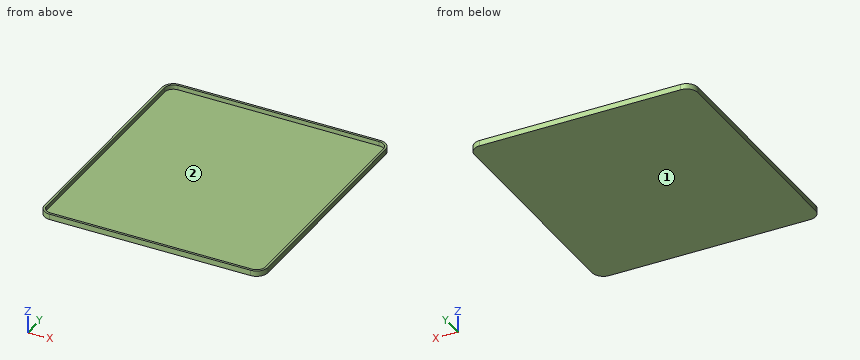
from build123d import *

# Parameters (mm, degrees)
F1_DEPTH = 0.5
F3_DEPTH = 2


with BuildPart() as f1:
    # F0 (on Top) → F1 (new body)
    with BuildSketch(Plane.XY):
        with BuildLine():
            Line((-45, -53.918237), (45, -53.918237))
            ThreePointArc((45, -53.918237), (48.535534, -52.453771), (50, -48.918237))
            Line((50, -48.918237), (50, 51.081763))
            ThreePointArc((50, 51.081763), (48.535534, 54.617297), (45, 56.081763))
            Line((45, 56.081763), (-45, 56.081763))
            ThreePointArc((-45, 56.081763), (-48.535534, 54.617297), (-50, 51.081763))
            Line((-50, 51.081763), (-50, -48.918237))
            ThreePointArc((-50, -48.918237), (-48.535534, -52.453771), (-45, -53.918237))
        make_face()
    extrude(amount=F1_DEPTH)

    # F2 (on face) → F3 (join)
    with BuildSketch(Plane.XY.offset(0.5)):
        with BuildLine():
            ThreePointArc((45, -53.918237), (48.535534, -52.453771), (50, -48.918237))
            Line((50, -48.918237), (50, 51.081763))
            ThreePointArc((50, 51.081763), (48.535534, 54.617297), (45, 56.081763))
            Line((45, 56.081763), (-45, 56.081763))
            ThreePointArc((-45, 56.081763), (-48.535534, 54.617297), (-50, 51.081763))
            Line((-50, 51.081763), (-50, -48.918237))
            ThreePointArc((-50, -48.918237), (-48.535534, -52.453771), (-45, -53.918237))
            Line((-45, -53.918237), (45, -53.918237))
        make_face()
        with BuildLine():
            Line((49, 51.081763), (49, -48.918237))
            ThreePointArc((49, -48.918237), (47.828427, -51.746664), (45, -52.918237))
            Line((45, -52.918237), (-45, -52.918237))
            ThreePointArc((-45, -52.918237), (-47.828427, -51.746664), (-49, -48.918237))
            Line((-49, -48.918237), (-49, 51.081763))
            ThreePointArc((-49, 51.081763), (-47.828427, 53.91019), (-45, 55.081763))
            Line((-45, 55.081763), (45, 55.081763))
            ThreePointArc((45, 55.081763), (47.828427, 53.91019), (49, 51.081763))
        make_face(mode=Mode.SUBTRACT)
    extrude(amount=F3_DEPTH)


solid = f1.part
Geometry check sheet. Reference: the model listing, model coordinates, mm. Face numbers are marked on the shaded views. Round coordinates to 2 decimals unless told otherwise and drop trailing zeros. Order: outer loops, then holes, each group sorted by start corner. A loop starts at its lowest first (then second) coordinate and runs counter-clockwise, first axis right, second up. Notation, with made-up numbers: M -14.5,25 L -9.5,25 A23 cw -9.5,59 Z; hole C 58,-26.5 d4. An arc over 180 degrees is marked long. Answer in a Markdown table with one row per item.
(1) Scan lines: probe 1 along X at (y, z) = (23, 1.5); probe 2 along Y at (x, z) = (-30.5, 1.4); probe 3 along Z at (x, y) = (18, 40). Record each from-to range of solid material in increasing order. Write a range as from..to.
Responses:
| item | result |
|---|---|
| probe 1 | x = -50..-49, 49..50 |
| probe 2 | y = -53.92..-52.92, 55.08..56.08 |
| probe 3 | z = 0..0.5 |
(2) Sectioned sample at A-A, the plane z = 1.9. Record the cut outline in (x, y), and give its area (3 significant figures).
Responses:
| item | result |
|---|---|
| outline | M -50,-48.92 A5 ccw -45,-53.92 L 45,-53.92 A5 ccw 50,-48.92 L 50,51.08 A5 ccw 45,56.08 L -45,56.08 A5 ccw -50,51.08 Z; hole M -49,-48.92 A4 ccw -45,-52.92 L 45,-52.92 A4 ccw 49,-48.92 L 49,51.08 A4 ccw 45,55.08 L -45,55.08 A4 ccw -49,51.08 Z |
| area | 408 mm² |
(3) Sectioned sample at B-B, the plane y = 47.5. Record the cut outline in (x, z), and give its area (3 significant figures).
Responses:
| item | result |
|---|---|
| outline | M -50,0 L 50,0 L 50,2.5 L 49,2.5 L 49,0.5 L -49,0.5 L -49,2.5 L -50,2.5 Z |
| area | 54.0 mm² |
(4) Sectioned sample at C-C, the plane x = 17. Record the cut outline in (y, z), and give its area (3 significant figures).
Responses:
| item | result |
|---|---|
| outline | M -53.92,0 L 56.08,0 L 56.08,2.5 L 55.08,2.5 L 55.08,0.5 L -52.92,0.5 L -52.92,2.5 L -53.92,2.5 Z |
| area | 59.0 mm² |
(5) Draft check along Y on the marked faces 1 and 2. Enter one of: released by +Y, released by -Y, zero draft, split by the parting line, or undercut.
Responses:
| item | result |
|---|---|
| face 1 | zero draft |
| face 2 | undercut |
(6) Go/stop test with flat-tipped pins: P1, Ø4, axis at x = 29.5, y = 8, coming from the +Z side; P2, Ø12, axis at x = 40, y = -14.5, coming from the -Z side. Record where each tip stops, or that it passes through.
Responses:
| item | result |
|---|---|
| P1 | stops at z = 0.5 |
| P2 | stops at z = 0 |
